Read the model definition and answer for the solid it produces. Units are mm, in the model's axes. A direction names the side the tool comes from. Round coordinates to 2 decimals unless told otherwise and drop trailing zeros. Loops run counter-clockwise (first coordinate to the right, second up) from the corner with the lowest first, then second, coordinate; pieces in that order, holes last. Notation, with made-up numbers: M -22.75,37 L 18.25,37 A22 ccw 18.25,43 Z; hole C -36.75,-16 d10. An arc over 180 degrees is marked long. Answer as CSV lines item,"result".
```python
from build123d import *

# Parameters (mm, degrees)
BOSS_EXTRUDE1_DEPTH                                 = 78
BOSS_EXTRUDE2_DEPTH                                 = 5
CUT_EXTRUDE1_START                                  = -20
SKETCH4_W                                           = 8
SKETCH4_H                                           = 16
CUT_EXTRUDE1_DEPTH                                  = 36
SKETCH4_5_W                                         = 8
SKETCH4_5_H                                         = 12
CUT_EXTRUDE2_DEPTH                                  = 50
CSK_FOR_1_4_FLAT_HEAD_SOCKET_CAP_SCREW1_D           = 6.7564
CSK_FOR_1_4_FLAT_HEAD_SOCKET_CAP_SCREW1_CSINK_D     = 13.4874
CSK_FOR_1_4_FLAT_HEAD_SOCKET_CAP_SCREW1_CSINK_ANGLE = 82
FILLET1_R                                           = 3
FILLET2_R                                           = 6
FILLET4_R                                           = 8
FILLET3_R                                           = 2
FILLET5_R                                           = 1
CHAMFER1_SIZE                                       = 5
CHAMFER2_SIZE                                       = 2


with BuildPart() as part:
    # Sketch1 → Boss-Extrude1 (new body)
    with BuildSketch(Plane(origin=(0, 0, 0), x_dir=(1, 0, 0), z_dir=(0, 1, 0))):
        Polygon((0, 0), (-23, 0), (-23, -8), (-8, -8), (-8, -104), (173.5, -104), (173.5, -8), (188.5, -8), (188.5, 0), (165.5, 0), (165.5, -96), (0, -96), align=None)
    extrude(amount=BOSS_EXTRUDE1_DEPTH)

    # Sketch2 → Boss-Extrude2 (add)
    with BuildSketch(Plane.XZ):
        Polygon((-23, 0), (188.5, 0), (188.5, 8), (173.5, 8), (173.5, 104), (-8, 104), (-8, 8), (-23, 8), align=None)
    extrude(amount=BOSS_EXTRUDE2_DEPTH)

    # Sketch4 → Cut-Extrude1 (cut)
    with BuildSketch(Plane(origin=(0, 78, 0), x_dir=(1, 0, 0), z_dir=(0, 1, 0)).offset(CUT_EXTRUDE1_START)):
        with Locations((-4, -16)):
            Rectangle(SKETCH4_W, SKETCH4_H)
        with Locations((-4, -48)):
            Rectangle(SKETCH4_W, SKETCH4_H)
        with Locations((-4, -80)):
            Rectangle(SKETCH4_W, SKETCH4_H)
    extrude(amount=-CUT_EXTRUDE1_DEPTH, mode=Mode.SUBTRACT)

    # Sketch4<5> → Cut-Extrude2 (cut)
    with BuildSketch(Plane(origin=(0, 78, 0), x_dir=(1, 0, 0), z_dir=(0, 1, 0))):
        with Locations((169.5, -48)):
            Rectangle(SKETCH4_5_W, SKETCH4_5_H)
        with Locations((169.5, -80)):
            Rectangle(SKETCH4_5_W, SKETCH4_5_H)
        with Locations((169.5, -16)):
            Rectangle(SKETCH4_5_W, SKETCH4_5_H)
    extrude(amount=-CUT_EXTRUDE2_DEPTH, mode=Mode.SUBTRACT)

    # CSK for 1/4 Flat Head Socket Cap Screw1 (through all)
    with Locations(Plane.XY.offset(8)):
        with Locations((181, 10), (181, 63)):
            csk_for_1_4_flat_head_socket_cap_screw1 = CounterSinkHole(CSK_FOR_1_4_FLAT_HEAD_SOCKET_CAP_SCREW1_D / 2, CSK_FOR_1_4_FLAT_HEAD_SOCKET_CAP_SCREW1_CSINK_D / 2, counter_sink_angle=CSK_FOR_1_4_FLAT_HEAD_SOCKET_CAP_SCREW1_CSINK_ANGLE)

    # Mirror1: CSK for 1/4 Flat Head Socket Cap Screw1 across plane
    add(csk_for_1_4_flat_head_socket_cap_screw1.mirror(Plane(origin=(82.75, 0, 0), x_dir=(0, 0, 1), z_dir=(1, 0, 0))), mode=Mode.SUBTRACT)

    # Fillet1
    fillet1_edges = [part.edges().sort_by_distance(p)[0] for p in [
        (-4, 22, 24),
        (-4, 22, 8),
        (-4, 58, 8),
        (-4, 58, 24),
        (-4, 58, 56),
        (-4, 58, 40),
        (-4, 22, 56),
        (-4, 22, 40),
        (-4, 58, 88),
        (-4, 58, 72),
        (-4, 22, 88),
        (-4, 22, 72),
    ]]
    fillet(fillet1_edges, radius=FILLET1_R)

    # Fillet2
    fillet2_edges = [part.edges().sort_by_distance(p)[0] for p in [
        (169.5, 28, 74),
        (169.5, 28, 42),
        (169.5, 28, 86),
        (169.5, 28, 54),
        (169.5, 28, 22),
        (169.5, 28, 10),
    ]]
    fillet(fillet2_edges, radius=FILLET2_R - 0.0001)  # a hair under: the kernel refuses the full size

    # Fillet4
    fillet4_edges = [part.edges().sort_by_distance(p)[0] for p in [
        (165.5, 0, 48),
        (0, 0, 48),
    ]]
    fillet(fillet4_edges, radius=FILLET4_R)

    # Fillet3
    fillet3_edges = [part.edges().sort_by_distance(p)[0] for p in [
        (165.5, 43, 0),
        (0, 43, 0),
        (82.75, 0, 0),
        (2.343145751, 2.343145751, 0),
        (163.156854249, 2.343145751, 0),
    ]]
    fillet(fillet3_edges, radius=FILLET3_R)

    # Fillet5
    fillet5_edges = [part.edges().sort_by_distance(p)[0] for p in [
        (0, 43, 96),
        (165.5, 43, 96),
        (82.75, 0, 96),
        (163.156854249, 2.343145751, 96),
        (2.343145751, 2.343145751, 96),
    ]]
    fillet(fillet5_edges, radius=FILLET5_R)

    # Chamfer1
    chamfer1_edges = [part.edges().sort_by_distance(p)[0] for p in [
        (-23, 78, 4),
        (173.5, 36.5, 104),
        (-8, 36.5, 104),
        (188.5, 78, 4),
        (-23, -5, 4),
        (188.5, -5, 4),
    ]]
    chamfer(chamfer1_edges, length=CHAMFER1_SIZE)

    # Chamfer2
    chamfer2_edges = [part.edges().sort_by_distance(p)[0] for p in [
        (82.75, -5, 0),
        (178.5, -5, 8),
        (173.5, -5, 53.5),
        (171, -5, 101.5),
        (82.75, -5, 104),
        (-5.5, -5, 101.5),
        (-13, -5, 8),
        (-8, -5, 53.5),
        (173.5, 78, 9),
        (178.5, 78, 8),
        (173.5, 78, 32),
        (165.5, 78, 32),
        (165.5, 78, 64),
        (173.5, 78, 64),
        (165.5, 78, 6),
        (175.5, 78, 0),
        (173.5, 78, 92.5),
        (171, 78, 101.5),
        (82.75, 78, 104),
        (-5.5, 78, 101.5),
        (-8, 78, 53.5),
        (-13, 78, 8),
        (165.5, 78, 90.5),
        (82.75, 78, 96),
        (-10, 78, 0),
        (0, 78, 48.5),
        (169.5, 78, 22),
        (169.5, 78, 42),
        (169.5, 78, 54),
        (169.5, 78, 74),
        (169.5, 78, 10),
        (169.5, 78, 86),
        (166.085786438, 78, 0.585786438),
        (-0.585786438, 78, 0.585786438),
        (165.207106781, 78, 95.707106781),
        (0.292893219, 78, 95.707106781),
    ]]
    chamfer(chamfer2_edges, length=CHAMFER2_SIZE - 0.0001)  # a hair under: the kernel refuses the full size


solid = part.part
```
1) Find section A-A, the plane x = -15.5. Give the vertices of the cut face in (y, z).
Evaluation:
outline,"M -5,2 L -3,0 L 6.62,0 L 6.62,4.13 L 3.26,8 L -3,8 L -5,6 Z; M 13.38,0 L 59.62,0 L 59.62,4.13 L 56.26,8 L 16.74,8 L 13.38,4.13 Z; M 66.38,0 L 76,0 L 78,2 L 78,6 L 76,8 L 69.74,8 L 66.38,4.13 Z"
2) Each of these flat-tipped pins is pushed along its axis until it touches: P1, Ø2.5, axis at x = 171, y = 50.5, coming from the +Z side; P2, Ø3, axis at y = 25, z = 46.5, coming from the -X side; P3, Ø12, axis at y = 6, z = 38.5, coming from the +X side; P4, Ø9, axis at x = 181, y = 63, coming from the -Z side. Where does it stop, or does it pass through?
Evaluation:
P1,"stops at z = 102.75"
P2,"stops at x = 165.5"
P3,"stops at x = 173.5"
P4,"stops at z = 0"
3) Determine the mould class of faces 4 (the flat face through (186, 75.5, 4.1)), 5 (the cylindrical face through (-13.941, 60.003, 2.035)), 6 (the flat face through (84, 37, 104)) for opening direction X: released by +X, released by -X, zero draft, split by the parting line, or undercut.
Evaluation:
face 4,"released by +X"
face 5,"undercut"
face 6,"zero draft"
4) Find section D-D, the plane x = 55. Give the vertices of the cut face in (y, z).
Evaluation:
outline,"M -5,2 L -3,0 L -2,0 A2 ccw 0,2 L 0,95 A1 cw 1,96 L 76,96 L 78,98 L 78,102 L 76,104 L -3,104 L -5,102 Z"
5) Straight lines are drawn through the part: line 1 (Y direction, x = 181, z = 2.25); line 2 (X direction, y = 10, z = 2); line 3 (X direction, y = 71, z = 90). For each, find the intervals that lie inside material, in ascending order.
Evaluation:
line 1,"y = -5 to 6.62, 13.38 to 59.62, 66.38 to 78"
line 2,"x = -23 to -18.88, -12.12 to 0, 165.5 to 177.62, 184.38 to 188.5"
line 3,"x = -8 to 0, 165.5 to 173.5"
6) A tool of negligible diameter and unlimited length cuts with its end or side. For faces 1 (the cylindrical face through (169.556, 29.804, 84.289)), 2 (the flat face through (169, 55, 54)), 3 (the flat face through (-4, 58, 16)), from which of +Z, -Z, +X, -X, +Y, -Y can it reach the whole face along a straight path? Write none if from no direction.
Evaluation:
face 1,"+X, -X, +Y"
face 2,"+X, +Y"
face 3,"+X, -X"
7) Find section B-B, the plane y = 10. Count the separate pieces of the cut face and the enclosed holes in it, then the cut area to 3 significant figures.
Evaluation:
separate pieces,"3"
enclosed holes,"0"
area,"3,070 mm^2"
8) Find section C-C, the plane z = 82. Give the vertices of the cut face in (x, y), then the cut area to 3 significant figures.
Evaluation:
outline,"M -8,-3 L -6,-5 L 171.5,-5 L 173.5,-3 L 173.5,28.34 L 165.5,28.34 L 165.5,8 A8 cw 157.5,0 L 8,0 A8 cw 0,8 L 0,22 L -8,22 Z; M -8,58 L 0,58 L 0,76 L -2,78 L -6,78 L -8,76 Z"
area,"1,490 mm^2"
